Verification items for the finished model (mm, model axes). A direction names the side the tool comes from. Give positions to 0.01 mm unless a question says otherwise; leave off trailing zeros. Write each loop counter-clockwise with the first axis right and the second up, starting at its lowest first coordinate (ties: lowest second). Pieces come first, ordered by that corner, then holes.
from build123d import *

# Parameters (mm, degrees)
BOSS_EXTRUDE1_DEPTH                                 = 12.7
CSK_FOR_1_4_FLAT_HEAD_MACHINE_SCREW_100_D           = 6.7564
CSK_FOR_1_4_FLAT_HEAD_MACHINE_SCREW_100_CSINK_D     = 12.8778
CSK_FOR_1_4_FLAT_HEAD_MACHINE_SCREW_100_CSINK_ANGLE = 100
SKETCH6_W                                           = 19.05
SKETCH6_H                                           = 15.875
BOSS_EXTRUDE2_DEPTH                                 = 9.0424
CSK_FOR_1_4_FLAT_HEAD_MACHINE_SCREW_2_D             = 6.7564
CSK_FOR_1_4_FLAT_HEAD_MACHINE_SCREW_2_CSINK_D       = 12.8778
CSK_FOR_1_4_FLAT_HEAD_MACHINE_SCREW_2_CSINK_ANGLE   = 100
CHAMFER1_SIZE                                       = 0.79375


with BuildPart() as part:
    # Sketch1 → Boss-Extrude1 (new body)
    with BuildSketch(Plane.XY):
        Polygon((-28.575, 19.05), (28.575, 19.05), (28.575, 3.175), (19.05, 3.175), (9.525, 3.175), (9.525, -19.05), (-9.525, -19.05), (-9.525, 3.175), (-19.05, 3.175), (-28.575, 3.175), align=None)
    extrude(amount=-BOSS_EXTRUDE1_DEPTH)

    # CSK for 1_4 Flat Head Machine Screw _100 (through all)
    with Locations(Plane.XY):
        with Locations((0, 10.16), (0, -10.16)):
            CounterSinkHole(CSK_FOR_1_4_FLAT_HEAD_MACHINE_SCREW_100_D / 2, CSK_FOR_1_4_FLAT_HEAD_MACHINE_SCREW_100_CSINK_D / 2, counter_sink_angle=CSK_FOR_1_4_FLAT_HEAD_MACHINE_SCREW_100_CSINK_ANGLE)

    # Sketch6 → Boss-Extrude2 (add)
    with BuildSketch(Plane.XY.offset(-12.7)):
        with Locations((-19.05, 11.1125)):
            Rectangle(SKETCH6_W, SKETCH6_H)
        with Locations((19.05, 11.1125)):
            Rectangle(SKETCH6_W, SKETCH6_H)
    extrude(amount=-BOSS_EXTRUDE2_DEPTH)

    # CSK for 1_4 Flat Head Machine Screw  2 (through all)
    with Locations(Plane(origin=(0, 19.05, 0), x_dir=(1, 0, 0), z_dir=(0, 1, 0))):
        with Locations((-19.05, 9.525), (19.05, 9.525)):
            CounterSinkHole(CSK_FOR_1_4_FLAT_HEAD_MACHINE_SCREW_2_D / 2, CSK_FOR_1_4_FLAT_HEAD_MACHINE_SCREW_2_CSINK_D / 2, counter_sink_angle=CSK_FOR_1_4_FLAT_HEAD_MACHINE_SCREW_2_CSINK_ANGLE)

    # Chamfer1
    chamfer1_edges = [part.edges().sort_by_distance(p)[0] for p in [
        (-9.525, 11.1125, -21.7424),
        (9.525, 11.1125, -21.7424),
    ]]
    chamfer(chamfer1_edges, length=CHAMFER1_SIZE)


solid = part.part
Item 1: Sectioned sample at B-B on x = 0. Record the cut outline in (y, z), then the cut area to 3 significant figures.
Answer key:
outline: (-19.05, -12.7) - (-13.54, -12.7) - (-13.54, -2.57) - (-16.6, 0) - (-19.05, 0) - close; (-6.78, -12.7) - (6.78, -12.7) - (6.78, -2.57) - (3.72, 0) - (-3.72, 0) - (-6.78, -2.57) - close; (13.54, -12.7) - (19.05, -12.7) - (19.05, 0) - (16.6, 0) - (13.54, -2.57) - close
area: 297 mm2
Item 2: Sectioned sample at A-A on y = 10.16. Record the cut outline in (x, z) (3 decimals).
Answer key:
outline: (-28.575, -21.742) - (-10.319, -21.742) - (-9.525, -20.949) - (-9.525, -12.7) - (-3.378, -12.7) - (-3.378, -2.568) - (-6.439, 0) - (-28.575, 0) - close; (3.378, -12.7) - (9.525, -12.7) - (9.525, -20.949) - (10.319, -21.742) - (28.575, -21.742) - (28.575, 0) - (6.439, 0) - (3.378, -2.568) - close; hole circle Ø6.756 at (-19.05, -9.525); hole circle Ø6.756 at (19.05, -9.525)
Item 3: Sectioned sample at C-C on y = -10.16. Record the cut outline in (x, z) (3 decimals).
Answer key:
outline: (-9.525, -12.7) - (-3.378, -12.7) - (-3.378, -2.568) - (-6.439, 0) - (-9.525, 0) - close; (3.378, -12.7) - (9.525, -12.7) - (9.525, 0) - (6.439, 0) - (3.378, -2.568) - close
Item 4: Depth check by flat-ended pin: pin 1 (12 mm diameter, centred on x = -16, z = -12.5, fed in from -Y) (3 decimals); pin 2 (5.5 mm diameter, centred on x = 19.05, z = -9.525, fed in from +Y); pin 3 (11 mm diameter, centred on x = 0, y = 10.16, fed in from -Z); pin 4 (10 mm diameter, centred on y = -12, z = -8, fed in from -X) (3 decimals). Enter the tip coordinate at first touch or a pass-through.
Answer key:
pin 1: stops at y = 3.175
pin 2: passes through
pin 3: stops at z = -12.7
pin 4: stops at x = -9.525
Item 5: Sectioned sample at D-D on x = 19.05. Record the cut outline in (y, z) (3 decimals).
Answer key:
outline: (3.175, -21.742) - (19.05, -21.742) - (19.05, -15.964) - (16.482, -12.903) - (3.175, -12.903) - close; (3.175, -6.147) - (16.482, -6.147) - (19.05, -3.086) - (19.05, 0) - (3.175, 0) - close
Item 6: Set-up check for faces 1 (the face through (0, 0, -12.7)), 2 (the face through (9.525, -8, -6)), 3 (the face through (0.765, 6.717, -2.444)): record each of +Z, -Z, +X, -X, +Y, -Y from which the full face is reachable in a straight line by a thin tool's end or side.
Answer key:
face 1: -Z, +Y, -Y
face 2: +Z, -Z, +X, -Y
face 3: +Z
Item 7: Release check for a two-part mould opening along X. For faces 4 (the face through (0, 19.05, -11)), 5 (the face through (-9.525, -8, -6)), 6 (the face through (-9.525, 11, -17)) record: released by +X, released by -X, zero draft, split by the parting line, or undercut.
Answer key:
face 4: zero draft
face 5: released by -X
face 6: undercut
Item 8: Scan lines: line 1 along Z through (x, y) = (19.05, 11.5); line 2 along X through (y, z) = (10.5, -20.5) (3 decimals); line 3 along X through (y, z) = (10.5, -12.25) (3 decimals). Record each from-to range of solid material in increasing order.
Answer key:
line 1: z = -21.74 to -12.9, -6.15 to 0
line 2: x = -28.575 to -9.525, 9.525 to 28.575
line 3: x = -28.575 to -21.047, -17.053 to -3.361, 3.361 to 17.053, 21.047 to 28.575
